The model under review builds one solid part; all positions refer to its coordinate system, in mm. A direction names the side the tool comes from. Coordinates: 2 decimals unless noted, no trailing zeros. Loops run counter-clockwise (first coordinate to the right, second up) from the corner with the lowest first, then second, coordinate; pieces in that order, holes last. Notation, with made-up numbers: (-15, -34.75) - (20, -34.75) arc R16 ccw to (20, -6.75) - close; hole circle Ø9 at (87.25, -37). An arc over 180 degrees is marked (long way). Use a Markdown table: item, result. Add a question column.
1) Add section A-A, the plane z = 1.5. Give the boundary of the cut face in (x, y), and give its area (3 significant figures).
2) For faces 1 (the flat face through (0.2, 7.7, -1.55)), 2 (the flat face through (1, -11.5, 2)), 3 (the flat face through (-1, -7.5, 2)), list the 3-axis set-ups (+Z, -Z, +X, -X, +Y, -Y) from which the entire face can be reached by the end or side of a thin tool; tool diameter is ignored.
3) Add section B-B, the plane y = 0. Give the number of separate pieces and of enclosed holes in the cut face, and give its area (3 significant figures).
4) Add section D-D, the plane y = 6.5. Give the boundary of the cut face in (x, z).
5) Add section C-C, the plane x = -23.5. Give the boundary of the cut face in (y, z).
6) To check wall thickness, follow L1, parallel to X at y = -6.5, z = -2.5; L2, parallel to Y at x = -27, z = 1; L3, parallel to Y at x = -40.8, z = 1.5. State the ranges of each line that lie inside material, in increasing order. Write a range as [from, to].
7) Clearance check with flat-ended pins moving along their axes: pin 1 (1.7 mm diameter, centred on y = 1, z = -1, fed in from +X); pin 2 (4 mm diameter, centred on x = 14.5, y = 6, fed in from -Z); pin 3 (1.2 mm diameter, centred on y = 0, z = 1.5, fed in from +X). State where each tip first meets the part, or that it passes through.
8) The part is to be moulded in two halves that separate along Z. For faces 4 (the flat face through (-1, 0, 3)), 5 (the flat face through (0.2, 7.7, -2)), 6 (the flat face through (1, 11.5, 2)), say which applies: pulls with the +Z half, pulls with the -Z half, needs draft (parallel to the pull), parting line crosses it, or undercut.
```python
from build123d import *

# Parameters (mm, degrees)
SKETCH1_W               = 76.5
SKETCH1_H               = 15
BOSS_EXTRUDE1_DEPTH     = 3
SKETCH2_R               = 1
CUT_EXTRUDE1_DEPTH      = 77.92528843
SKETCH3_W               = 84.5
SKETCH3_H               = 23
BOSS_EXTRUDE2_DEPTH     = 7
CUT_EXTRUDE2_DEPTH      = 82.618012718
CUT_EXTRUDE2_DEPTH_BACK = 82.618012718
SKETCH4_R               = 1
SKETCH5_W               = 77.5
SKETCH5_H               = 16
SKETCH5_W_2             = 76.5
SKETCH5_H_2             = 15
CUT_EXTRUDE4_DEPTH      = 0.48
SKETCH10_W              = 84.5
SKETCH10_H              = 23
SKETCH10_W_2            = 76.5
SKETCH10_H_2            = 15
BOSS_EXTRUDE7_DEPTH     = 2
SKETCH11_W              = 77.5
SKETCH11_H              = 16
SKETCH11_W_2            = 76.5
SKETCH11_H_2            = 15
CUT_EXTRUDE5_DEPTH      = 0.45
SKETCH13_W              = 84.5
SKETCH13_H              = 23
SKETCH13_W_2            = 76.5
SKETCH13_H_2            = 15
BOSS_EXTRUDE8_DEPTH     = 2
CUT_EXTRUDE6_START      = -4.48
CUT_EXTRUDE6_DEPTH      = 4.48


with BuildPart() as part:
    # Sketch1 → Boss-Extrude1 (new body)
    with BuildSketch(Plane.XY):
        Rectangle(SKETCH1_W, SKETCH1_H)
    extrude(amount=BOSS_EXTRUDE1_DEPTH)

    # Sketch2 → Cut-Extrude1 (cut, through all)
    with BuildSketch(Plane(origin=(38.25, 0, 0), x_dir=(0, 0, -1), z_dir=(1, 0, 0))):
        with Locations((-1.5, 0)):
            Circle(SKETCH2_R)
    extrude(amount=-CUT_EXTRUDE1_DEPTH, mode=Mode.SUBTRACT)


with BuildPart() as body_2:
    # Sketch3 → Boss-Extrude2 (new body)
    with BuildSketch(Plane(origin=(0, 0, 0), x_dir=(-1, 0, 0), z_dir=(0, 0, -1))):
        Rectangle(SKETCH3_W, SKETCH3_H)
    extrude(amount=-BOSS_EXTRUDE2_DEPTH)

    # Combine1: cut part
    add(part.part, mode=Mode.SUBTRACT)

    # Sketch4 → Cut-Extrude2 (cut, two sides: drawn at the far end of the back side and taken through both)
    with BuildSketch(Plane.ZY.offset(-38.25).offset(-CUT_EXTRUDE2_DEPTH_BACK)):
        with Locations((1.5, 0)):
            Circle(SKETCH4_R)
    extrude(amount=CUT_EXTRUDE2_DEPTH + CUT_EXTRUDE2_DEPTH_BACK, mode=Mode.SUBTRACT)

    # Sketch5 → Cut-Extrude4 (cut)
    with BuildSketch(Plane(origin=(0, 0, 0), x_dir=(-1, 0, 0), z_dir=(0, 0, -1))):
        Rectangle(SKETCH5_W, SKETCH5_H)
        Rectangle(SKETCH5_W_2, SKETCH5_H_2, mode=Mode.SUBTRACT)
    extrude(amount=-CUT_EXTRUDE4_DEPTH, mode=Mode.SUBTRACT)

    # Sketch10 → Boss-Extrude7 (add)
    with BuildSketch(Plane(origin=(0, 0, 0), x_dir=(-1, 0, 0), z_dir=(0, 0, -1))):
        Rectangle(SKETCH10_W, SKETCH10_H)
        Rectangle(SKETCH10_W_2, SKETCH10_H_2, mode=Mode.SUBTRACT)
    extrude(amount=BOSS_EXTRUDE7_DEPTH)

    # Sketch11 → Cut-Extrude5 (cut)
    with BuildSketch(Plane(origin=(0, 0, -2), x_dir=(-1, 0, 0), z_dir=(0, 0, -1))):
        Rectangle(SKETCH11_W, SKETCH11_H)
        Rectangle(SKETCH11_W_2, SKETCH11_H_2, mode=Mode.SUBTRACT)
    extrude(amount=-CUT_EXTRUDE5_DEPTH, mode=Mode.SUBTRACT)

    # Sketch13 → Boss-Extrude8 (add)
    with BuildSketch(Plane(origin=(0, 0, -2), x_dir=(-1, 0, 0), z_dir=(0, 0, -1))):
        Rectangle(SKETCH13_W, SKETCH13_H)
        Rectangle(SKETCH13_W_2, SKETCH13_H_2, mode=Mode.SUBTRACT)
    extrude(amount=BOSS_EXTRUDE8_DEPTH)

    # Sketch14 → Cut-Extrude6 (cut)
    with BuildSketch(Plane(origin=(0, 0, -4), x_dir=(-1, 0, 0), z_dir=(0, 0, -1)).offset(CUT_EXTRUDE6_START)):
        Polygon((-42.25, -5), (-38.25, -2.5), (-38.25, 2.5), (-42.25, 5), align=None)
    extrude(amount=CUT_EXTRUDE6_DEPTH, mode=Mode.SUBTRACT)


solid = body_2.part
```
From the geometry:
| question | item | result |
|---|---|---|
| 1 | outline | (-42.25, -11.5) - (42.25, -11.5) - (42.25, -1) - (38.25, -1) - (38.25, -7.5) - (-38.25, -7.5) - (-38.25, -1) - (-42.25, -1) - close; (-42.25, 1) - (-38.25, 1) - (-38.25, 7.5) - (38.25, 7.5) - (38.25, 1) - (42.25, 1) - (42.25, 11.5) - (-42.25, 11.5) - close |
| 1 | area | 780 mm^2 |
| 2 | face 1 | none |
| 2 | face 2 | +Z, -Z, +X, -X, -Y |
| 2 | face 3 | -Z |
| 3 | separate pieces | 3 |
| 3 | enclosed holes | 0 |
| 3 | area | 360 mm^2 |
| 4 | outline | (-42.25, -4) - (-38.25, -4) - (-38.25, -2) - (-38.75, -2) - (-38.75, -1.55) - (-38.25, -1.55) - (-38.25, 0) - (-38.75, 0) - (-38.75, 0.48) - (-38.25, 0.48) - (-38.25, 3) - (38.25, 3) - (38.25, 0.48) - (38.75, 0.48) - (38.75, 0) - (38.25, 0) - (38.25, -1.55) - (38.75, -1.55) - (38.75, -2) - (38.25, -2) - (38.25, -4) - (42.25, -4) - (42.25, 7) - (-42.25, 7) - close |
| 5 | outline | (-11.5, -4) - (-7.5, -4) - (-7.5, -2) - (-8, -2) - (-8, -1.55) - (-7.5, -1.55) - (-7.5, 0) - (-8, 0) - (-8, 0.48) - (-7.5, 0.48) - (-7.5, 3) - (7.5, 3) - (7.5, 0.48) - (8, 0.48) - (8, 0) - (7.5, 0) - (7.5, -1.55) - (8, -1.55) - (8, -2) - (7.5, -2) - (7.5, -4) - (11.5, -4) - (11.5, 7) - (-11.5, 7) - close |
| 6 | L1 | x = [-42.25, -38.25], [38.25, 42.25] |
| 6 | L2 | y = [-11.5, -7.5], [7.5, 11.5] |
| 6 | L3 | y = [-11.5, -1], [1, 11.5] |
| 7 | pin 1 | stops at x = -38.25 |
| 7 | pin 2 | stops at z = -4 |
| 7 | pin 3 | passes through |
| 8 | face 4 | pulls with the -Z half |
| 8 | face 5 | undercut |
| 8 | face 6 | needs draft |
